from build123d import *

# Parameters (mm, degrees)
SKETCH1_R           = 1
SKETCH1_W           = 8.8
SKETCH1_H           = 4
BOSS_EXTRUDE1_DEPTH = 0.5
SKETCH2_W           = 15.5
SKETCH2_H           = 0.65
BOSS_EXTRUDE2_DEPTH = 5.7
SKETCH5_W           = 2
SKETCH5_H           = 0.65
BOSS_EXTRUDE4_DEPTH = 1
SKETCH6_W           = 1
SKETCH6_H           = 0.5
BOSS_EXTRUDE5_DEPTH = 1.5
FILLET1_R           = 0.5
SKETCH7_W           = 1
SKETCH7_H           = 0.5
BOSS_EXTRUDE6_DEPTH = 1.5
FILLET2_R           = 0.5


with BuildPart() as part:
    # Sketch1 → Boss-Extrude1 (new body)
    with BuildSketch(Plane(origin=(0, 0, 0), x_dir=(1, 0, 0), z_dir=(0, 1, 0))):
        with BuildLine():
            Line((11.6, 2.6), (11.6, -2.6))
            ThreePointArc((11.6, -2.6), (11.453553391, -2.953553391), (11.1, -3.1))
            Line((11.1, -3.1), (7.75, -3.1))
            Line((7.75, -3.1), (7.75, -3.75))
            Line((7.75, -3.75), (-7.75, -3.75))
            Line((-7.75, -3.75), (-7.75, -3.1))
            Line((-7.75, -3.1), (-11.1, -3.1))
            ThreePointArc((-11.1, -3.1), (-11.453553391, -2.953553391), (-11.6, -2.6))
            Line((-11.6, -2.6), (-11.6, 2.6))
            ThreePointArc((-11.6, 2.6), (-11.453553391, 2.953553391), (-11.1, 3.1))
            Line((-11.1, 3.1), (-7.75, 3.1))
            Line((-7.75, 3.1), (-7.75, 3.75))
            Line((-7.75, 3.75), (7.75, 3.75))
            Line((7.75, 3.75), (7.75, 3.1))
            Line((7.75, 3.1), (11.1, 3.1))
            ThreePointArc((11.1, 3.1), (11.453553391, 2.953553391), (11.6, 2.6))
        make_face()
        with Locations((9.5, 0)):
            Circle(SKETCH1_R, mode=Mode.SUBTRACT)
        with Locations((-9.5, 0)):
            Circle(SKETCH1_R, mode=Mode.SUBTRACT)
        Rectangle(SKETCH1_W, SKETCH1_H, mode=Mode.SUBTRACT)
    extrude(amount=-BOSS_EXTRUDE1_DEPTH)

    # Sketch2 → Boss-Extrude2 (add)
    with BuildSketch(Plane.XZ.offset(0.5)):
        with Locations((0, 3.425)):
            Rectangle(SKETCH2_W, SKETCH2_H)
        with Locations((0, -3.425)):
            Rectangle(SKETCH2_W, SKETCH2_H)
    extrude(amount=BOSS_EXTRUDE2_DEPTH)

    # Sketch5 → Boss-Extrude4 (add)
    with BuildSketch(Plane.XZ.offset(6.2)):
        with Locations((-5.75, 3.425)):
            Rectangle(SKETCH5_W, SKETCH5_H)
        with Locations((-5.75, -3.425)):
            Rectangle(SKETCH5_W, SKETCH5_H)
        with Locations((5.75, -3.425)):
            Rectangle(SKETCH5_W, SKETCH5_H)
        with Locations((5.75, 3.425)):
            Rectangle(SKETCH5_W, SKETCH5_H)
    extrude(amount=BOSS_EXTRUDE4_DEPTH)

    # Sketch6 → Boss-Extrude5 (add)
    with BuildSketch(Plane(origin=(0, 0, -3.75), x_dir=(-1, 0, 0), z_dir=(0, 0, -1))):
        with Locations((-6.25, -7.45)):
            Rectangle(SKETCH6_W, SKETCH6_H)
        with Locations((6.25, -7.45)):
            Rectangle(SKETCH6_W, SKETCH6_H)
    extrude(amount=-BOSS_EXTRUDE5_DEPTH)

    # Fillet1
    fillet1_edges = [part.edges().sort_by_distance(p)[0] for p in [
        (-6.25, -7.7, -3.75),
        (6.25, -7.7, -3.75),
        (0, 0, -3.75),
    ]]
    fillet(fillet1_edges, radius=FILLET1_R)

    # Sketch7 → Boss-Extrude6 (add)
    with BuildSketch(Plane.XY.offset(3.75)):
        with Locations((-6.25, -7.45)):
            Rectangle(SKETCH7_W, SKETCH7_H)
        with Locations((6.25, -7.45)):
            Rectangle(SKETCH7_W, SKETCH7_H)
    extrude(amount=-BOSS_EXTRUDE6_DEPTH)

    # Fillet2
    fillet2_edges = [part.edges().sort_by_distance(p)[0] for p in [
        (0, 0, 3.75),
        (6.25, -7.7, 3.75),
        (-6.25, -7.7, 3.75),
    ]]
    fillet(fillet2_edges, radius=FILLET2_R)


solid = part.part
The model under review builds one solid part; all positions refer to its coordinate system, in mm. A direction names the side the tool comes from. Round coordinates to 2 decimals unless told otherwise and drop trailing zeros. Order: outer loops, then holes, each group sorted by start corner. A loop starts at its lowest first (then second) coordinate and runs counter-clockwise, first axis right, second up. Notation, with made-up numbers: (70, 85.25) -> (82, 85.25) arc R26 ccw to (82, 115.25) -> close; hole circle Ø10 at (85, 12). An arc over 180 degrees is marked (long way). Return JSON: item names as keys, results as strings.
1. Take a section at D-D (x = 5). Write out the cut boundary in (y, z).
Answer block:
{"outline": "(-7.2, -3.75) -> (-0.5, -3.75) arc R0.5 ccw to (0, -3.25) -> (0, 3.25) arc R0.5 ccw to (-0.5, 3.75) -> (-7.2, 3.75) -> (-7.2, 3.1) -> (-0.5, 3.1) -> (-0.5, -3.1) -> (-7.2, -3.1) -> close"}
2. Insertion check: P1, Ø3, axis at x = 8, z = -2, coming from the +Y side; P2, Ø1, axis at x = 2.5, z = 2.5, coming from the -Y side; P3, Ø2, axis at y = -6, z = -3, coming from the -X side; P4, Ø0.5, axis at x = 7.5, z = 3.5, coming from the -Y side. Each pin has a flat end and moves straight along its axis. Give the tip position at first contact, or say it passes through.
Answer block:
{"P1": "stops at y = 0", "P2": "stops at y = -0.5", "P3": "stops at x = -7.75", "P4": "stops at y = -6.2"}
3. For faces 5 (the face through (-6.75, -7.1, -3.3)), 6 (the face through (6.75, -7.1, -3.3)), 7 (the face through (6.3, -7.2, -2.7)), 8 (the face through (0.2, 0, -2.2)), list the 3-axis set-ups (+Z, -Z, +X, -X, +Y, -Y) from which the entire face can be reached by the end or side of a thin tool; tool diameter is ignored.
Answer block:
{"face 5": "+Z, -Z, -X, -Y", "face 6": "+Z, -Z, +X, -Y", "face 7": "+X, -X", "face 8": "+Z, -Z, +X, -X, +Y"}
4. Take a section at B-B (x = 9.5). Write out the cut boundary in (y, z).
Answer block:
{"outline": "(-0.5, -3.1) -> (0, -3.1) -> (0, -1) -> (-0.5, -1) -> close; (-0.5, 1) -> (0, 1) -> (0, 3.1) -> (-0.5, 3.1) -> close"}
5. For L1, parallel to X at y = -0.4, z = 0; L2, parallel to Z at x = -1, y = -3; L3, parallel to Z at x = 9.5, y = -0.25, list the stretches that pass through material, from the lowest coordinate up. Write a range as [from, to].
Answer block:
{"L1": "x = [-11.6, -10.5], [-8.5, -4.4], [4.4, 8.5], [10.5, 11.6]", "L2": "z = [-3.75, -3.1], [3.1, 3.75]", "L3": "z = [-3.1, -1], [1, 3.1]"}
6. The part is to be moulded in two halves that separate along Y. For faces 1 (the face through (6.2, -7.2, 2.7)), 2 (the face through (-6.2, -7.2, -2.7)), 3 (the face through (6.75, -7.1, 3.3)), 4 (the face through (-6, -7.7, -3)), say which applies: +Y half, -Y half, draft (parallel to the pull), parting line (faces both ways), or undercut.
Answer block:
{"face 1": "undercut", "face 2": "undercut", "face 3": "draft", "face 4": "-Y half"}
7. Take a section at C-C (z = 0). Write out the cut boundary in (x, y).
Answer block:
{"outline": "(-11.6, -0.5) -> (-10.5, -0.5) -> (-10.5, 0) -> (-11.6, 0) -> close; (-8.5, -0.5) -> (-4.4, -0.5) -> (-4.4, 0) -> (-8.5, 0) -> close; (4.4, -0.5) -> (8.5, -0.5) -> (8.5, 0) -> (4.4, 0) -> close; (10.5, -0.5) -> (11.6, -0.5) -> (11.6, 0) -> (10.5, 0) -> close"}
8. Take a section at A-A (y = -5.75). Write out the cut boundary in (x, z), then the cut area to 4 significant figures.
Answer block:
{"outline": "(-7.75, -3.75) -> (7.75, -3.75) -> (7.75, -3.1) -> (-7.75, -3.1) -> close; (-7.75, 3.1) -> (7.75, 3.1) -> (7.75, 3.75) -> (-7.75, 3.75) -> close", "area": "20.15 mm²"}
